```python
from build123d import *

# Parameters (mm, degrees)
SKETCH_1_W                                   = 56
SKETCH_1_H                                   = 8
FOOT_56X24X8_DEPTH                           = 24
SKETCH_2_W                                   = 44
SKETCH_2_H                                   = 74
TOWER_PIVOT_HEIGHT60_DEPTH                   = 8
SHAFT_ACCESS_AND_RETAINER_M3_DEPTH           = 83.680106434
SHAFT_ACCESS_AND_RETAINER_M3_DEPTH_BACK      = 83.680106434
SKETCH_3_R                                   = 5.8
SKETCH_3_R_2                                 = 1.7
SKETCH_4_R                                   = 8.1
F_625ZZ_POCKET_D16P2_DEPTH5P2_TEST_FIT_DEPTH = 5.2
FOOT_M3_THROUGH_DEPTH                        = 83.680106434
FOOT_M3_THROUGH_DEPTH_BACK                   = 83.680106434
SKETCH_5_R                                   = 1.7


with BuildPart() as part:
    # 草图1 → Foot_56x24x8 (new body)
    with BuildSketch(Plane.XY):
        with Locations((0, 4)):
            Rectangle(SKETCH_1_W, SKETCH_1_H)
    extrude(amount=FOOT_56X24X8_DEPTH)

    # 草图2 → Tower_pivot_height60 (add)
    with BuildSketch(Plane.XY):
        with Locations((0, 37)):
            Rectangle(SKETCH_2_W, SKETCH_2_H)
    extrude(amount=TOWER_PIVOT_HEIGHT60_DEPTH)

    # 草图3 → Shaft_access_and_retainer_M3 (cut, two sides: drawn at the far end of the back side and taken through both)
    with BuildSketch(Plane.XY.offset(-SHAFT_ACCESS_AND_RETAINER_M3_DEPTH_BACK)):
        with Locations((0, 60)):
            Circle(SKETCH_3_R)
        with Locations((-14, 60)):
            Circle(SKETCH_3_R_2)
        with Locations((14, 60)):
            Circle(SKETCH_3_R_2)
    extrude(amount=SHAFT_ACCESS_AND_RETAINER_M3_DEPTH + SHAFT_ACCESS_AND_RETAINER_M3_DEPTH_BACK, mode=Mode.SUBTRACT)

    # 草图4 → 625ZZ_pocket_D16p2_depth5p2_TEST_FIT (cut)
    with BuildSketch(Plane.XY):
        with Locations((0, 60)):
            Circle(SKETCH_4_R)
    extrude(amount=F_625ZZ_POCKET_D16P2_DEPTH5P2_TEST_FIT_DEPTH, mode=Mode.SUBTRACT)

    # 草图5 → Foot_M3_through (cut, two sides: drawn at the far end of the back side and taken through both)
    with BuildSketch(Plane(origin=(0, 0, 0), x_dir=(1, 0, 0), z_dir=(0, 1, 0)).offset(-FOOT_M3_THROUGH_DEPTH_BACK)):
        with Locations(Location((-20, -12, 0), (0, 0, 270))):
            Circle(SKETCH_5_R)
        with Locations(Location((20, -12, 0), (0, 0, 270))):
            Circle(SKETCH_5_R)
    extrude(amount=FOOT_M3_THROUGH_DEPTH + FOOT_M3_THROUGH_DEPTH_BACK, mode=Mode.SUBTRACT)


solid = part.part
```
Could you check a few things on this model? Use its own coordinates, in mm. A direction names the side the tool comes from. Round coordinates to 2 decimals unless told otherwise and drop trailing zeros. Loops run counter-clockwise (first coordinate to the right, second up) from the corner with the lowest first, then second, coordinate; pieces in that order, holes last. Notation, with made-up numbers: M 7,85 L 45,85 A33 ccw 45,118 Z; hole C -29.5,16.25 d2. An arc over 180 degrees is marked long. Write item = value, one per line.
1. I want a section at C-C, the plane z = 21.25. Write out the boundary of the cut face in (x, y).
Results below:
outline = M -28,0 L 28,0 L 28,8 L -28,8 Z
2. Which directions (+Z, -Z, +X, -X, +Y, -Y) give clear straight access to the entire face, cutting with the end or side of a thin tool? Please do faces 4 (the face through (-2, 66, 5.2)), 5 (the face through (22, 41, 4)), 6 (the face through (-22, 41, 4)).
Results below:
face_4 = -Z
face_5 = +Z, -Z, +X, +Y
face_6 = +Z, -Z, -X, +Y
3. Will these pins go through, and if not, where does the flat tip stop? P1, Ø22, axis at x = -3, y = 34.5, coming from the +Z side; P2, Ø9, axis at y = 36.5, z = 5.5, coming from the +X side; P3, Ø4.5, axis at x = 20, z = 12, coming from the +Y side.
Results below:
P1 = 8
P2 = 22
P3 = 8
4. I need wall thicknesses on probe 1 along X at (y, z) = (2, 12); probe 2 along X at (y, z) = (60, 6); probe 3 along Y at (x, z) = (-14, 5.25). Which ranges of each line are inside material? Lowest first, please.
Results below:
probe_1 = -28 to -21.7, -18.3 to 18.3, 21.7 to 28
probe_2 = -22 to -15.7, -12.3 to -5.8, 5.8 to 12.3, 15.7 to 22
probe_3 = 0 to 58.3, 61.7 to 74
5. I want a section at A-A, the plane y = 60. Write out the boundary of the cut face in (x, z).
Results below:
outline = M -22,0 L -15.7,0 L -15.7,8 L -22,8 Z; M -12.3,0 L -8.1,0 L -8.1,5.2 L -5.8,5.2 L -5.8,8 L -12.3,8 Z; M 5.8,5.2 L 8.1,5.2 L 8.1,0 L 12.3,0 L 12.3,8 L 5.8,8 Z; M 15.7,0 L 22,0 L 22,8 L 15.7,8 Z
6. I want a section at B-B, the plane x = 0. Write out the boundary of the cut face in (y, z), and give its area (3 significant figures).
Results below:
outline = M 0,0 L 51.9,0 L 51.9,5.2 L 54.2,5.2 L 54.2,8 L 8,8 L 8,24 L 0,24 Z; M 65.8,5.2 L 68.1,5.2 L 68.1,0 L 74,0 L 74,8 L 65.8,8 Z
area = 603 mm²
7. Thinking about a two-plate mould opening in Z: for faces 1 (the face through (-0.76, 65.75, 6.58)), 2 (the face through (-18.567, 3.944, 12.914)), 3 (the face through (0, 4, 24)), which applies, +Z half, -Z half, draft (parallel to the pull), parting line (faces both ways), or undercut?
Results below:
face_1 = draft
face_2 = undercut
face_3 = +Z half
8. I want a section at D-D, the plane x = 20. Write out the boundary of the cut face in (y, z).
Results below:
outline = M 0,0 L 74,0 L 74,8 L 8,8 L 8,10.3 L 0,10.3 Z; M 0,13.7 L 8,13.7 L 8,24 L 0,24 Z
